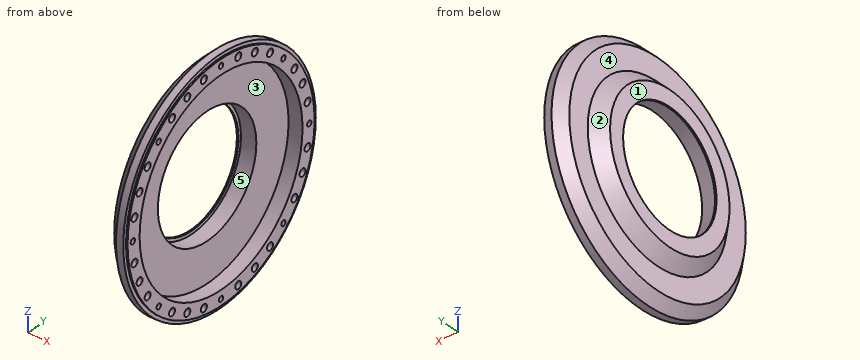
from build123d import *

# Parameters (mm, degrees)
SKETCH5_R          = 2.38125
CUT_EXTRUDE1_DEPTH = 4.445
SKETCH6_R          = 1.7272
CUT_EXTRUDE2_DEPTH = 9.525


with BuildPart() as part:
    # Sketch4 → Revolve1 (revolve)
    with BuildSketch(Plane.XY):
        Polygon((7.249924984, 74.025000032), (6.249924952, 74.025000032), (6.249924952, 76.2), (1.53480008, 76.2), (-4.81519992, 69.85), (-4.81519992, 55.24999999), (-12.775199748, 47.290000162), (-12.775199748, 36.999999914), (-11.775199716, 36.999999914), (-11.775199716, 38.999999978), (-1.815199824, 38.999999978), (-1.815199824, 64.500000032), (7.249924984, 64.500000032), align=None)
    revolve(axis=Axis((0, 0, 0), (1, 0, 0)))

    # Sketch5 → Cut-Extrude1 (cut)
    with BuildSketch(Plane(origin=(7.249924984, 0, 0), x_dir=(0, 0, -1), z_dir=(1, 0, 0))):
        with Locations((13.627058993, 68.507851836)):
            Circle(SKETCH5_R)
        with Locations((26.730437751, 64.532985346)):
            Circle(SKETCH5_R)
        with Locations((38.806580776, 58.078152419)):
            Circle(SKETCH5_R)
        with Locations((58.078152419, 38.806580776)):
            Circle(SKETCH5_R)
        with Locations((64.532985346, 26.730437751)):
            Circle(SKETCH5_R)
        with Locations((68.507851836, 13.627058993)):
            Circle(SKETCH5_R)
        with Locations((68.507851836, -13.627058993)):
            Circle(SKETCH5_R)
        with Locations((64.532985346, -26.730437751)):
            Circle(SKETCH5_R)
        with Locations((58.078152419, -38.806580776)):
            Circle(SKETCH5_R)
        with Locations((38.806580776, -58.078152419)):
            Circle(SKETCH5_R)
        with Locations((26.730437751, -64.532985346)):
            Circle(SKETCH5_R)
        with Locations((13.627058993, -68.507851836)):
            Circle(SKETCH5_R)
        with Locations((-13.627058993, -68.507851836)):
            Circle(SKETCH5_R)
        with Locations((-26.730437751, -64.532985346)):
            Circle(SKETCH5_R)
        with Locations((-38.806580776, -58.078152419)):
            Circle(SKETCH5_R)
        with Locations((-58.078152419, -38.806580776)):
            Circle(SKETCH5_R)
        with Locations((-64.532985346, -26.730437751)):
            Circle(SKETCH5_R)
        with Locations((-68.507851836, -13.627058993)):
            Circle(SKETCH5_R)
        with Locations((-68.507851836, 13.627058993)):
            Circle(SKETCH5_R)
        with Locations((-64.532985346, 26.730437751)):
            Circle(SKETCH5_R)
        with Locations((-58.078152419, 38.806580776)):
            Circle(SKETCH5_R)
        with Locations((-38.806580776, 58.078152419)):
            Circle(SKETCH5_R)
        with Locations((-26.730437751, 64.532985346)):
            Circle(SKETCH5_R)
        with Locations((-13.627058993, 68.507851836)):
            Circle(SKETCH5_R)
    extrude(amount=-CUT_EXTRUDE1_DEPTH, mode=Mode.SUBTRACT)

    # Sketch6 → Cut-Extrude2 (cut)
    with BuildSketch(Plane(origin=(7.249924984, 0, 0), x_dir=(0, 0, -1), z_dir=(1, 0, 0))):
        with Locations((0, 69.85)):
            Circle(SKETCH6_R)
        with Locations((-49.391408666, 49.391408666)):
            Circle(SKETCH6_R)
        with Locations((-69.85, 0)):
            Circle(SKETCH6_R)
        with Locations((-49.391408666, -49.391408666)):
            Circle(SKETCH6_R)
        with Locations((0, -69.85)):
            Circle(SKETCH6_R)
        with Locations((49.391408666, -49.391408666)):
            Circle(SKETCH6_R)
        with Locations((69.85, 0)):
            Circle(SKETCH6_R)
        with Locations((49.391408666, 49.391408666)):
            Circle(SKETCH6_R)
    extrude(amount=-CUT_EXTRUDE2_DEPTH, mode=Mode.SUBTRACT)


solid = part.part
Can you work these out from the model? Positions are in its coordinate system, mm. Face numbers are marked on the shaded views. A direction names the side the tool comes from. Coordinates: 2 decimals unless noted, no trailing zeros. Loops run counter-clockwise (first coordinate to the right, second up) from the corner with the lowest first, then second, coordinate; pieces in that order, holes last. Notation, with made-up numbers: M 28.5,-15 L 54.5,-15 A20 cw 54.5,9 Z; hole C -36,-13 d2. An arc over 180 degrees is marked long. Return JSON: item names as keys, results as strings. Group by question number.
Item 1: On a 3-axis mill with a long thin cutter (end or side, diameter ignored), from which of +Z, -Z, +X, -X, +Y, -Y can I reach the whole of each face in a straight line? I mean the marked faces 4 and 5. Say none if no direction works.
Item 2: I'm going to push flat-ended pins straight in: pin 1 Ø3 at (x, y) = (0, 37) entering from -Z; pin 2 Ø1.5 at (x, y) = (-1.5, -51) entering from -Z; pin 3 Ø2 at (x, y) = (-9, 30.5) entering from -Z. Where does each tip first touch, or does it pass through?
Item 3: Thinking about a two-plate mould opening in Z: for the marked faces 1, 2 and 3, which applies, released by +Z, released by -Z, zero draft, split by the parting line, or undercut?
Item 4: Imagine slicing it at A-A (x = -10). Please give me the cut outline in (y, z), and give its area (3 significant figures).
Item 5: If I drill on L1, parallel to Z at x = 4.75, y = -41; L2, parallel to Y at x = -10.75, z = -14; L3, parallel to X at y = -11.5, z = 36.5, over which ranges is the centre line in solid material (lowest first)? Write a range as from..to.
Verdict:
{
 "1": {"face 4": "-X", "face 5": "+X"},
 "2": {"pin 1": "stops at z = -66.76", "pin 2": "stops at z = -53.72", "pin 3": "stops at z = -42.39"},
 "3": {"face 1": "zero draft", "face 2": "split by the parting line", "face 3": "undercut"},
 "4": {"outline": "C 0,0 d100.13; hole C 0,0 d78", "area": "3,100 mm^2"},
 "5": {"L1": "z = -64.23..-59.01, -57.15..-49.79, 49.79..57.15, 59.01..64.23", "L2": "y = -47.29..-36.4, 36.4..47.29", "L3": "x = -12.78..-11.78"}
}
